Input: dimensioned drawing with shaded views. Units: mm. Origin: part minimum x, y, z. Give positions to 0.01 mm unless a question says otherwise; leave off trailing zeros. Write each loop counter-clockwise with the first axis right and the second up, starting at its lowest first coordinate (ties: lowest second). Pieces come first, ordered by that corner, then holes. Notation, with made-up numbers: (15.5, -17.5) -> (45.5, -17.5) arc R20 ccw to (45.5, -9.5) -> close; hole circle Ø3 at (55.25, -34.75). An arc over 180 degrees is marked (long way). Answer as a JSON object with one key per item and string values. Group by question number.
(1) Section query D-D on y = 69. Output: boundary loops of the cut face in (x, z), plus the area to 3 significant figures.
(2) Section query A-A on y = 92. Output: boundary loops of the cut face in (x, z), plus the area to 3 significant figures.
(3) Material intervals for probe 1 along Y at (x, z) = (92, 1.7); probe 2 along X at (y, z) = (21.5, 1.3), sorted ascending.
(4) Contact query for flat-ended pins moving along their axis: pin 1 Ø4.5 at (x, y) = (92, 92) entering from -Z; pin 2 Ø3 at (x, y) = (92, 4) entering from -Z. Output: stop coordinate, or through.
(5) Section query C-C on x = 48. Output: boundary loops of the cut face in (y, z).
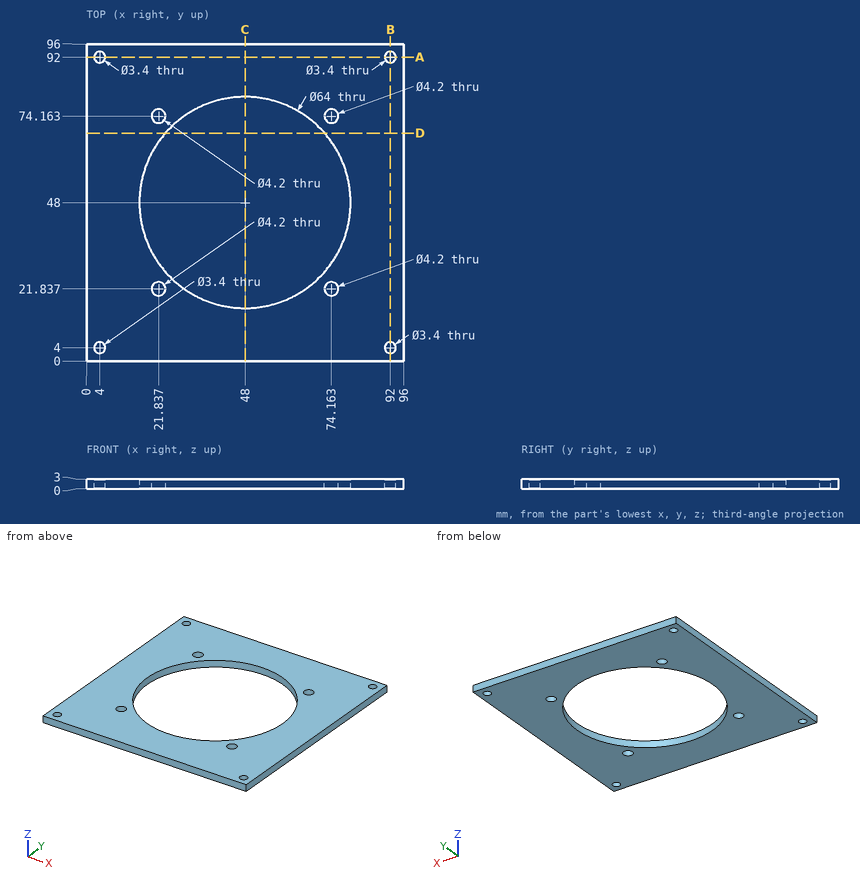
Answer list:
{
 "1": {"outline": "(0, 0) -> (23.85, 0) -> (23.85, 3) -> (0, 3) -> close; (72.15, 0) -> (96, 0) -> (96, 3) -> (72.15, 3) -> close", "area": "143 mm2"},
 "2": {"outline": "(0, 0) -> (2.3, 0) -> (2.3, 3) -> (0, 3) -> close; (5.7, 0) -> (90.3, 0) -> (90.3, 3) -> (5.7, 3) -> close; (93.7, 0) -> (96, 0) -> (96, 3) -> (93.7, 3) -> close", "area": "268 mm2"},
 "3": {"probe 1": "0 to 2.3, 5.7 to 90.3, 93.7 to 96", "probe 2": "0 to 19.76, 23.91 to 30.06, 65.94 to 72.09, 76.24 to 96"},
 "4": {"pin 1": "z = 0", "pin 2": "through"},
 "5": {"outline": "(0, 0) -> (16, 0) -> (16, 3) -> (0, 3) -> close; (80, 0) -> (96, 0) -> (96, 3) -> (80, 3) -> close"}
}
